```python
from build123d import *

# Parameters (mm, degrees)
F0_R            = 34.925
F1_DEPTH        = 6.35
F3_D            = 4.9784
F3_COPIES_COUNT = 6
F5_D            = 8.334375


# Not quite as in the source:
# - a pattern or mirror of a feature is missing from the dataset's text; its kind, count and spacing are read off the source's solid


with BuildPart() as f1:
    # F0 (on Top) → F1 (new body)
    with BuildSketch(Plane.XY):
        Circle(F0_R)
    extrude(amount=F1_DEPTH)

    # F3 (through all)
    with Locations(Plane.XY.offset(6.35)):
        with Locations((0, 28.575)):
            f3 = Hole(F3_D / 2)

    # F3_copies: F3 ×6 about axis
    f3_copies_axis = Axis((0, 0, 0), (0, 0, 1))
    for i in range(1, F3_COPIES_COUNT):
        add(f3.rotate(f3_copies_axis, i * 360 / F3_COPIES_COUNT), mode=Mode.SUBTRACT)

    # F5 (through all)
    with Locations(Plane.XY.offset(6.35)):
        with Locations((0, 0)):
            Hole(F5_D / 2)


solid = f1.part
```
Here's how the part is built. I have some questions about the finished solid (model axes, mm). Round coordinates to 2 decimals unless told otherwise and drop trailing zeros. Write each loop counter-clockwise with the first axis right and the second up, starting at its lowest first coordinate (ties: lowest second). Pieces come first, ordered by that corner, then holes.
Q1. If we section it at C-C on z = 3.25: Give the number of separate pieces and of enclosed holes in the cut face, plus the area to 3 significant figures.
Q2. If we section it at B-B on x = 0: Write out the boundary of the cut face in (y, z) (3 decimals), plus the area to 3 significant figures.
Q3. Will these pins go through, and if not, where does the flat tip stop? P1, Ø1.5, axis at x = 3, z = 3, coming from the -Y side; P2, Ø2, axis at y = 15, z = 4.5, coming from the -X side; P3, Ø1, axis at x = -18.5, z = 2, coming from the -Y side.
Q4. If we section it at D-D on y = 27.5: Write out the boundary of the cut face in (x, z), plus the area to 3 significant figures.
Q5. Please list where these lines run through material, in increasing order: probe 1 along Y at (x, z) = (0, 4.25) (3 decimals); probe 2 along Y at (x, z) = (-1.5, 1.25); probe 3 along X at (y, z) = (14.5, 1.5).
Q6. If we section it at A-A on y = 0: Write out the boundary of the cut face in (x, z) (3 decimals).
Q7. If we mould it in two halves opening along Y, with no side actions, what happens to faces 1 (the flat face through (7, 0, 0)), 2 (the cylindrical face through (-22.26, -14.18, 3.13)), 3 (the cylindrical face through (-27.715, -21.251, 3.131))? For each: +Y half, -Y half, draft (parallel to the pull), parting line (faces both ways), or undercut.
Answer below:
1. separate pieces: 1
1. enclosed holes: 7
1. area: 3,660 mm2
2. outline: (-34.925, 0) - (-31.064, 0) - (-31.064, 6.35) - (-34.925, 6.35) - close; (-26.086, 0) - (-4.167, 0) - (-4.167, 6.35) - (-26.086, 6.35) - close; (4.167, 0) - (26.086, 0) - (26.086, 6.35) - (4.167, 6.35) - close; (31.064, 0) - (34.925, 0) - (34.925, 6.35) - (31.064, 6.35) - close
2. area: 327 mm2
3. P1: stops at y = -34.85
3. P2: stops at x = -32
3. P3: stops at y = -29.93
4. outline: (-21.53, 0) - (-2.25, 0) - (-2.25, 6.35) - (-21.53, 6.35) - close; (2.25, 0) - (21.53, 0) - (21.53, 6.35) - (2.25, 6.35) - close
4. area: 245 mm2
5. probe 1: y = -34.925 to -31.064, -26.086 to -4.167, 4.167 to 26.086, 31.064 to 34.925
5. probe 2: y = -34.89 to -30.56, -26.59 to -3.89, 3.89 to 26.59, 30.56 to 34.89
5. probe 3: x = -31.77 to -27.23, -22.27 to 22.27, 27.23 to 31.77
6. outline: (-34.925, 0) - (-4.167, 0) - (-4.167, 6.35) - (-34.925, 6.35) - close; (4.167, 0) - (34.925, 0) - (34.925, 6.35) - (4.167, 6.35) - close
7. face 1: draft
7. face 2: undercut
7. face 3: parting line
